```python
from build123d import *

# Parameters (mm, degrees)
SKETCH3_R           = 5
SKETCH1_R           = 8
SKETCH4_R           = 5
BOSS_EXTRUDE1_DEPTH = 5
BOSS_EXTRUDE1_TAPER = -15
SKETCH5_R           = 5
BOSS_EXTRUDE2_DEPTH = 20


with BuildPart() as part:
    # Sketch3 → Loft1 section 0
    with BuildSketch(Plane(origin=(0, 7, 0), x_dir=(1, 0, 0), z_dir=(0, 1, 0))):
        Circle(SKETCH3_R)
    # Sketch1 → Loft1 section 1
    with BuildSketch(Plane(origin=(0, 0, 0), x_dir=(1, 0, 0), z_dir=(0, 1, 0))):
        Circle(SKETCH1_R)
    loft()

    # Sketch4 → Boss-Extrude1 (add)
    with BuildSketch(Plane(origin=(0, -5, 0), x_dir=(-1, 0, 0), z_dir=(0, -1, 0))):
        Circle(SKETCH4_R)
    extrude(amount=-BOSS_EXTRUDE1_DEPTH, taper=BOSS_EXTRUDE1_TAPER)

    # Sketch5 → Boss-Extrude2 (add)
    with BuildSketch(Plane(origin=(0, -5, 0), x_dir=(-1, 0, 0), z_dir=(0, -1, 0))):
        Circle(SKETCH5_R)
    extrude(amount=BOSS_EXTRUDE2_DEPTH)


solid = part.part
```
Verification items for the finished model (mm, model axes). A direction names the side the tool comes from. Give positions to 0.01 mm unless a question says otherwise; leave off trailing zeros. Order: outer loops, then holes, each group sorted by start corner. A loop starts at its lowest first (then second) coordinate and runs counter-clockwise, first axis right, second up. Notation, with made-up numbers: M -0.5,74 L 35.5,74 A13 ccw 35.5,80 Z; hole C 58,79.5 d8. An arc over 180 degrees is marked long. Answer in a Markdown table with one row per item. Add a question column.
Item 1: Section check A-A, the plane x = 0. Enter the section's corners in (y, z).
Item 2: Section check B-B, the plane y = -15.5. Enter the section's corners in (x, z).
Item 3: Scan lines: probe 1 along Z at (x, y) = (-4.5, -7); probe 2 along X at (y, z) = (-10.5, 1.5); probe 3 along Z at (x, y) = (-0.75, -7). Record each from-to range of solid material in increasing order. Write a range as from..to.
Item 4: Section check C-C, the plane y = -1.5. Enter the section's corners in (x, z).
Item 5: Mould release check, pull along Y, two halves, no side actions. Record for faces 3 (the flat face through (0, 7, 0)), 4 (the cylindrical face through (1.08, -14.86, 4.88)), 5 (the flat face through (0, -25, 0)): released by +Y, released by -Y, zero draft, split by the parting line, or undercut.
Item 6: Tool access check on faces 1 (the conical face through (5.1, 5.8, 2.1)), 2 (the flat face through (-5.4, 0, -3.6)). Record the directions out of +Z, -Z, +X, -X, +Y, -Y that give a thin tool (end or side, any length) a straight path to the whole face; none if there is none.
Item 7: Gauge pin test, flat ends, axial feed: pin 1 (1 mm diameter, centred on x = -5, z = -3.5, fed in from +Y); pin 2 (8 mm diameter, centred on y = -6.5, z = -1, fed in from -X); pin 3 (2 mm diameter, centred on x = -4, z = 5, fed in from +Y). Record the tip position at first contact, or that the pin passes through.
Filled sheet:
| question | item | result |
|---|---|---|
| 1 | outline | M -25,-5 L -5,-5 L 0,-6.34 L 0,-8 L 7,-5 L 7,5 L 0,8 L 0,6.34 L -5,5 L -25,5 Z |
| 2 | outline | C 0,0 d10 |
| 3 | probe 1 | z = -2.18..2.18 |
| 3 | probe 2 | x = -4.77..4.77 |
| 3 | probe 3 | z = -4.94..4.94 |
| 4 | outline | C 0,0 d11.88 |
| 5 | face 3 | released by +Y |
| 5 | face 4 | zero draft |
| 5 | face 5 | released by -Y |
| 6 | face 1 | +Y |
| 6 | face 2 | -Y |
| 7 | pin 1 | stops at y = 5.59 |
| 7 | pin 2 | stops at x = -5.65 |
| 7 | pin 3 | stops at y = 6.06 |
